```python
from build123d import *

# Parameters (mm, degrees)
F1_DEPTH    = 10
F2_T1_DEPTH = 10
F2_T3_DEPTH = 85
F3_T        = -1


# Not quite as in the source:
# - a fillet or chamfer that OpenCascade refuses, or shapes differently, is made with other operations: its cross-section is extruded or revolved along the edge and cut away or added


with BuildPart() as f1:
    # F0 (on Top) → F1 (new body)
    with BuildSketch(Plane.XY):
        Polygon((0, 90), (0, 0), (30, 0), (30, 60), (57.2968044168, 60), (57.2968044168, 0), (90, 0), (90, 90), align=None)
    extrude(amount=F1_DEPTH)

    # F2: fillet of radius 15 on 8 edges, made by hand

    # F2_s2 → F2_t1 (join)
    with BuildSketch(Plane.XY):
        with BuildLine():
            ThreePointArc((42.2968044168, 60), (52.9034061346, 55.6066017178), (57.2968044168, 45))
            Line((57.2968044168, 45), (57.2968044168, 60))
            Line((57.2968044168, 60), (42.2968044168, 60))
        make_face()
        with BuildLine():
            ThreePointArc((30, 45), (34.3933982822, 55.6066017178), (45, 60))
            Line((45, 60), (30, 60))
            Line((30, 60), (30, 45))
        make_face()
    extrude(amount=F2_T1_DEPTH)

    # F2_s4 → F2_t3 (cut)
    with BuildSketch(Plane.XY.offset(-37.5)):
        with BuildLine():
            ThreePointArc((75, 90), (85.6066017178, 85.6066017178), (90, 75))
            Line((90, 75), (90, 90))
            Line((90, 90), (75, 90))
        make_face()
        with BuildLine():
            ThreePointArc((90, 15), (85.6066017178, 4.3933982822), (75, 0))
            Line((75, 0), (90, 0))
            Line((90, 0), (90, 15))
        make_face()
        with BuildLine():
            ThreePointArc((15, 0), (25.6066017178, 4.3933982822), (30, 15))
            Line((30, 15), (30, 0))
            Line((30, 0), (15, 0))
        make_face()
        with BuildLine():
            ThreePointArc((57.2968044168, 15), (61.690202699, 4.3933982822), (72.2968044168, 0))
            Line((72.2968044168, 0), (57.2968044168, 0))
            Line((57.2968044168, 0), (57.2968044168, 15))
        make_face()
        with BuildLine():
            ThreePointArc((0, 15), (4.3933982822, 4.3933982822), (15, 0))
            Line((15, 0), (0, 0))
            Line((0, 0), (0, 15))
        make_face()
        with BuildLine():
            ThreePointArc((0, 75), (4.3933982822, 85.6066017178), (15, 90))
            Line((15, 90), (0, 90))
            Line((0, 90), (0, 75))
        make_face()
    extrude(amount=F2_T3_DEPTH, mode=Mode.SUBTRACT)

    # F3
    f3_openings = [f1.faces().sort_by_distance(p)[0] for p in [
        (5.293398, 84.706602, 10),
    ]]
    offset(amount=F3_T, openings=f3_openings, kind=Kind.INTERSECTION)


solid = f1.part
```
The listing builds one solid part. Answer for the finished solid, in the listing's coordinates (mm). A direction names the side the tool comes from. Give positions to 0.01 mm unless a question says otherwise; leave off trailing zeros. Loops run counter-clockwise (first coordinate to the right, second up) from the corner with the lowest first, then second, coordinate; pieces in that order, holes last. Notation, with made-up numbers: M -36.5,49.5 L 7.5,49.5 A16 ccw 7.5,63.5 Z; hole C 84.5,82.25 d8. An arc over 180 degrees is marked long. One line per item, written item: value.
1. Section B-B on z = 4.75 is taken. Determine the outline of the cut face in (x, y).
Found:
outline: M 0,15 A15 ccw 30,15 L 30,45 A15 cw 43.65,59.94 A15 cw 57.3,45 L 57.3,15 A15 ccw 72.3,0 L 75,0 A15 ccw 90,15 L 90,75 A15 ccw 75,90 L 15,90 A15 ccw 0,75 Z; hole M 1,15 A14 ccw 29,15 L 29,45 A16 cw 43.65,60.94 A16 cw 58.3,45 L 58.3,15 A14 ccw 72.3,1 L 75,1 A14 ccw 89,15 L 89,75 A14 ccw 75,89 L 15,89 A14 ccw 1,75 Z
2. Each of these flat-tipped pins is pushed along its axis until it touches: P1, Ø10, axis at x = 52.5, y = 10.5, coming from the +Z side; P2, Ø4, axis at x = 60, z = 5, coming from the -Y side; P3, Ø4.5, axis at x = 47, z = 4.5, coming from the -Y side; P4, Ø3, axis at x = 79.5, z = 2.5, coming from the -Y side. Where does it stop, or does it pass through?
Found:
P1: through
P2: y = 4.09
P3: y = 58.29
P4: y = 0.3
3. Section D-D on y = 82.5 is taken. Determine the outline of the cut face in (x, z), plus the area to 3 significant figures.
Found:
outline: M 2.01,0 L 87.99,0 L 87.99,10 L 86.82,10 L 86.82,1 L 3.18,1 L 3.18,10 L 2.01,10 Z
area: 107 mm^2
4. For faces 4 (the face through (74, 1, 5)), 5 (the face through (33.82, 55, 4.93)), 6 (the face through (4.28, 85.49, 4.93)), determine the directions among +Z, -Z, +X, -X, +Y, -Y from which every point of the face is accessible in a straight line to the end or side of a thin tool.
Found:
face 4: +Z
face 5: +Z, -Z, -Y
face 6: +Z, -Z, -X, +Y
5. Section C-C on x = 31.5 is taken. Determine the outline of the cut face in (y, z).
Found:
outline: M 51.54,0 L 90,0 L 90,10 L 89,10 L 89,1 L 53.59,1 L 53.59,10 L 51.54,10 Z
6. Section A-A on y = 25 is taken. Determine the outline of the cut face in (x, z).
Found:
outline: M 0,0 L 30,0 L 30,10 L 29,10 L 29,1 L 1,1 L 1,10 L 0,10 Z; M 57.3,0 L 90,0 L 90,10 L 89,10 L 89,1 L 58.3,1 L 58.3,10 L 57.3,10 Z
7. Find the intervals of material crossed by probe 1 along X at (y, z) = (23.5, 5.25); probe 2 along X at (y, z) = (74.5, 7); probe 3 along X at (y, z) = (51, 9.25), in increasing order.
Found:
probe 1: 0 to 1, 29 to 30, 57.3 to 58.3, 89 to 90
probe 2: 0 to 1, 89 to 90
probe 3: 0 to 1, 30.17 to 31.25, 56.04 to 57.13, 89 to 90
8. For a pull along Y with two mould halves and no side action, classify faces 1 (the face through (45, 90, 5)), 2 (the face through (30, 30, 5)), 3 (the face through (53.965, 55.947, 5.437)) as pulls with the +Y half, pulls with the -Y half, needs draft (parallel to the pull), parting line crosses it, or undercut.
Found:
face 1: pulls with the +Y half
face 2: needs draft
face 3: undercut
